```python
from build123d import *

# Parameters (mm, degrees)
F0_W     = 60
F0_H     = 42
F1_DEPTH = 1.6
F2_R     = 11.5
F2_R_2   = 8.5
F3_DEPTH = 1.601
F5_DEPTH = 1.6
F6_R     = 3
F7_R     = 2
F8_W     = 22
F8_H     = 1.5
F9_DEPTH = 1.601
F10_R    = 1


with BuildPart() as f1:
    # F0 (on Top) → F1 (new body)
    with BuildSketch(Plane.XY):
        Rectangle(F0_W, F0_H)
    extrude(amount=F1_DEPTH)

    # F2 (on face) → F3 (cut, through all)
    with BuildSketch(Plane.XY.offset(1.6)):
        with Locations((14.7, 5.9)):
            Circle(F2_R)
        with Locations((-17, 7.25)):
            Circle(F2_R_2)
    extrude(amount=-F3_DEPTH, mode=Mode.SUBTRACT)

    # F4 (on Top) → F5 (join)
    with BuildSketch(Plane.XY):
        Polygon((-17.5, 25.4231041372), (-17.5, 20.9231041372), (-16, 20.9231041372), (-16, 23.9231041372), (6, 23.9231041372), (6, 20.9231041372), (7.5, 20.9231041372), (7.5, 25.4231041372), align=None)
    extrude(amount=F5_DEPTH)

    # F6
    f6_edges = [f1.edges().sort_by_distance(p)[0] for p in [
        (-30, 21, 0.8),
        (-30, -21, 0.8),
        (30, 21, 0.8),
        (30, -21, 0.8),
    ]]
    fillet(f6_edges, radius=F6_R)

    # F7
    f7_edges = [f1.edges().sort_by_distance(p)[0] for p in [
        (-17.5, 21, 0.8),
        (7.5, 21, 0.8),
    ]]
    fillet(f7_edges, radius=F7_R)

    # F8 (on face) → F9 (cut, through all)
    with BuildSketch(Plane.XY.offset(1.6)):
        with Locations((-5, 20.25)):
            Rectangle(F8_W, F8_H)
    extrude(amount=-F9_DEPTH, mode=Mode.SUBTRACT)

    # F10
    f10_edges = [f1.edges().sort_by_distance(p)[0] for p in [
        (-16, 23.923104, 0.8),
        (6, 23.923104, 0.8),
        (7.5, 25.423104, 0.8),
        (-17.5, 25.423104, 0.8),
        (-16, 19.5, 0.8),
        (6, 19.5, 0.8),
    ]]
    fillet(f10_edges, radius=F10_R)


solid = f1.part
```
Check sheet for the modelled part. Datum: model origin and axes. Units: mm. A direction names the side the tool comes from. Coordinates: 2 decimals unless noted, no trailing zeros. Write each loop counter-clockwise with the first axis right and the second up, starting at its lowest first coordinate (ties: lowest second). Pieces come first, ordered by that corner, then holes. Notation, with made-up numbers: M 65,-30 L 120,-30 A35 ccw 120,2 Z; hole C -25.5,-11 d11. An arc over 180 degrees is marked long. Write item = value, one per line. Start each with the question number.
1. Sectioned sample at A-A (x = -0.5). Record the cut outline in (y, z).
2. Go/stop test with flat-tipped pins: pin 1 (0.5 mm diameter, centred on y = 22.5, z = 0.5, fed in from -X); pin 2 (10 mm diameter, centred on x = 23, y = -9, fed in from -Z); pin 3 (0.5 mm diameter, centred on y = 22, z = 1, fed in from +X); pin 4 (0.5 mm diameter, centred on x = 18.5, z = 0.5, fed in from +Y). Record where each tip stops, or that it passes through.
3. Mould release check, pull along Y, two halves, no side actions. Record for faces 5 (the flat face through (-17.5, 24, 1)), 6 (the flat face through (-5, 25.423, 1)), 7 (the cylindrical face through (-18.84, -1.05, 0.81)): pulls with the +Y half, pulls with the -Y half, needs draft (parallel to the pull), parting line crosses it, or undercut.
4. Sectioned sample at B-B (z = 1). Record the cut outline in (x, y).
5. Sectioned sample at D-D (x = 14.7). Record the cut outline in (y, z).
6. Thickness scan on probe 1 along Y at (x, z) = (14.7, 0.3); probe 2 along X at (y, z) = (6.5, 0.5); probe 3 along Y at (x, z) = (-19, 0.35). Record the ranges inside material, lowest first.
7. Sectioned sample at C-C (y = 5.9). Record the cut outline in (x, z), then the cut area to 3 significant figures.
8. Tool access check on faces 1 (the flat face through (-5, 23.923, 1)), 2 (the flat face through (30, 0, 1)), 3 (the flat face through (-23, 21, 1)), 4 (the flat face through (18, 21, 1)). Record the directions out of +Z, -Z, +X, -X, +Y, -Y that give a thin tool (end or side, any length) a straight path to the whole face; none if there is none.
The answers:
q1.outline = M -21,0 L 19.5,0 L 19.5,1.6 L -21,1.6 Z; M 23.92,0 L 25.42,0 L 25.42,1.6 L 23.92,1.6 Z
q2.pin_1 = -17.65
q2.pin_2 = 0
q2.pin_3 = 7.94
q2.pin_4 = 21
q3.face_5 = needs draft
q3.face_6 = pulls with the +Y half
q3.face_7 = undercut
q4.outline = M -30,-18 A3 ccw -27,-21 L 27,-21 A3 ccw 30,-18 L 30,18 A3 ccw 27,21 L 9.5,21 A2 cw 7.5,23 L 7.5,24.42 A1 ccw 6.5,25.42 L -16.5,25.42 A1 ccw -17.5,24.42 L -17.5,23 A2 cw -19.5,21 L -27,21 A3 ccw -30,18 Z; hole C -17,7.25 d17; hole M -16,20.5 A1 ccw -15,19.5 L 5,19.5 A1 ccw 6,20.5 L 6,22.92 A1 ccw 5,23.92 L -15,23.92 A1 ccw -16,22.92 Z; hole C 14.7,5.9 d23
q5.outline = M -21,0 L -5.6,0 L -5.6,1.6 L -21,1.6 Z; M 17.4,0 L 21,0 L 21,1.6 L 17.4,1.6 Z
q6.probe_1 = -21 to -5.6, 17.4 to 21
q6.probe_2 = -30 to -25.47, -8.53 to 3.22, 26.18 to 30
q6.probe_3 = -21 to -1.01, 15.51 to 21.06
q7.outline = M -30,0 L -25.39,0 L -25.39,1.6 L -30,1.6 Z; M -8.61,0 L 3.2,0 L 3.2,1.6 L -8.61,1.6 Z; M 26.2,0 L 30,0 L 30,1.6 L 26.2,1.6 Z
q7.area = 32.3 mm²
q8.face_1 = +Z, -Z
q8.face_2 = +Z, -Z, +X, +Y, -Y
q8.face_3 = +Z, -Z, -X, +Y
q8.face_4 = +Z, -Z, +X, +Y
